Could you check a few things on this model? Use its own coordinates, in mm. A direction names the side the tool comes from. Give positions to 0.01 mm unless a question says otherwise; leave off trailing zeros. Order: outer loops, then holes, each group sorted by start corner. A loop starts at its lowest first (then second) coordinate and runs counter-clockwise, first axis right, second up.
Autodesk Inventor part; units mm, degrees
ref_plane "YZ Plane" through (0, 0, 0) normal (1, 0, 0) x (0, 1, 0)
ref_plane "XZ Plane" through (0, 0, 0) normal (0, 1, 0) x (-1, 0, 0)
ref_plane "XY Plane" through (0, 0, 0) normal (0, 0, 1) x (1, 0, 0)
sketch "草圖1" plane through (0, 0, 0) normal (0, 0, 1) x (1, 0, 0)
  line L0 (20, 0) -> (40, 0)
  line L1 (30, 50) -> (0, 50)
  line L2 (0, 50) -> (0, 20)
  arc A0 (0, 20) -> (20, 0) centre (20, 20) ccw
  line L3 (30, 50) -> (30, 40)
  line L4 (30, 40) -> (10, 40)
  line L5 (10, 40) -> (10, 20)
  arc A1 (10, 20) -> (20, 10) centre (20, 20) ccw
  line L6 (40, 10) -> (20, 10)
  line L7 (40, 0) -> (50, 0)
  line L8 (50, 0) -> (50, 10)
  line L9 (50, 10) -> (40, 10)
  point P0 (0, 0)
  dimension "d0" = 30
  dimension "d1" = 10
  dimension "d9" = 10
  dimension "d10" = 20
  dimension "d11" = 20
  dimension "d17" = 10
  dimension "d18" = 10
extrude "擠出1" add sketch "草圖1" along normal blind 40
sketch "草圖2" plane through (20, 10, 0) normal (0, 1, 0) x (1, 0, 0)
  circle A0 centre (10, -20) radius 10
  point P0 (-20, 0)
  dimension "d14" = 20
extrude "擠出2" cut sketch "草圖2" against normal blind 40
sketch "草圖3" plane through (20, 10, 0) normal (0, 1, 0) x (1, 0, 0)
  line L0 (30, 0) -> (0, 0)
  line L1 (30, 0) -> (30, -40)
  line L2 (30, -40) -> (0, -40)
  arc A0 (10, -40) -> (10, 0) centre (10, -20) ccw
  line L3 (10, -40) -> (30, -40)
  line L4 (30, -20) -> (30, 0)
  point P0 (-20, 0)
  dimension "d20" = 40
extrude "擠出3" cut sketch "草圖3" against normal blind 40
properties part number "40823233"
Item 1: Please list where these lines run through material, in increasing order: line 1 along Z through (x, y) = (30, 5); line 2 along Y through (x, z) = (19.5, 33.5); line 3 along X through (y, z) = (27, 34).
Findings:
line 1: z = 0 to 10, 30 to 40
line 2: y = 0.01 to 10.01, 40 to 50
line 3: x = 0 to 10
Item 2: Imagine slicing it at D-D on z = 31.5. List the corners of the cut face in (x, y) for me, then the cut area to 3 significant figures.
Findings:
outline: (0, 20) arc R20 ccw to (20, 0) - (46.36, 0) - (46.36, 10) - (20, 10) arc R10 cw to (10, 20) - (10, 40) - (30, 40) - (30, 50) - (0, 50) - close
area: 999 mm2
Item 3: Imagine slicing it at A-A on z = 23. List the corners of the cut face in (x, y) for me.
Findings:
outline: (0, 20) arc R20 ccw to (20, 0) - (20.46, 0) - (20.46, 10) - (20, 10) arc R10 cw to (10, 20) - (10, 40) - (30, 40) - (30, 50) - (0, 50) - close; (39.54, 0) - (49.77, 0) - (49.77, 10) - (39.54, 10) - close
Item 4: For pin 1 (5 mm diameter, centred on y = 43, z = 15.5, fed in from +X); pin 2 (1.5 mm diameter, centred on y = 18.5, z = 12.5, fed in from -X); pin 3 (12 mm diameter, centred on y = 8.5, z = 9, fed in from +X), each with a flat end and sliding along its axis, tell me the tip position at first contact or that it passes through.
Findings:
pin 1: stops at x = 30
pin 2: stops at x = 0.01
pin 3: stops at x = 49.36
Item 5: Imagine slicing it at C-C on z = 11. List the corners of the cut face in (x, y) for me.
Findings:
outline: (0, 20) arc R20 ccw to (20, 0) - (25.64, 0) - (25.64, 10) - (20, 10) arc R10 cw to (10, 20) - (10, 40) - (30, 40) - (30, 50) - (0, 50) - close; (34.36, 0) - (47.86, 0) - (47.86, 10) - (34.36, 10) - close
Item 6: Imagine slicing it at B-B on y = 46. List the corners of the cut face in (x, z) for me.
Findings:
outline: (0, 0) - (30, 0) - (30, 40) - (0, 40) - close
Item 7: For faces 4 (the cylindrical face through (39.54, 5.07, 17)), 5 (the flat face through (20, 40, 20)), 6 (the flat face through (41, 0, 20)), which set-ups out of +Z, -Z, +X, -X, +Y, -Y let a thin tool reach every point of the face, with its end or its side?
Findings:
face 4: -Y
face 5: +Z, -Z, +X
face 6: +Z, -Z, +X, -X, -Y
Item 8: We'd pull the mould along Y, two halves only. Please class faces 1 (the flat face through (10, 30, 20)), 2 (the flat face through (30, 45, 20)), 3 (the cylindrical face through (6.014, 5.703, 19.72)): +Y half, -Y half, draft (parallel to the pull), parting line (faces both ways), or undercut.
Findings:
face 1: undercut
face 2: draft
face 3: -Y half
